Input: dimensioned drawing with shaded views. Units: mm. Origin: part minimum x, y, z. A direction names the side the tool comes from. Round coordinates to 2 decimals unless told otherwise and drop trailing zeros. Loops run counter-clockwise (first coordinate to the right, second up) from the corner with the lowest first, then second, coordinate; pieces in that order, holes last. Notation, with made-up numbers: (65, -18) - (112, -18) arc R17 ccw to (112, 10) - close; hole circle Ø11 at (71, 55). An arc over 180 degrees is marked (long way). Use CSV: the item, a comma, the result in double quotes. Start each with the question number.
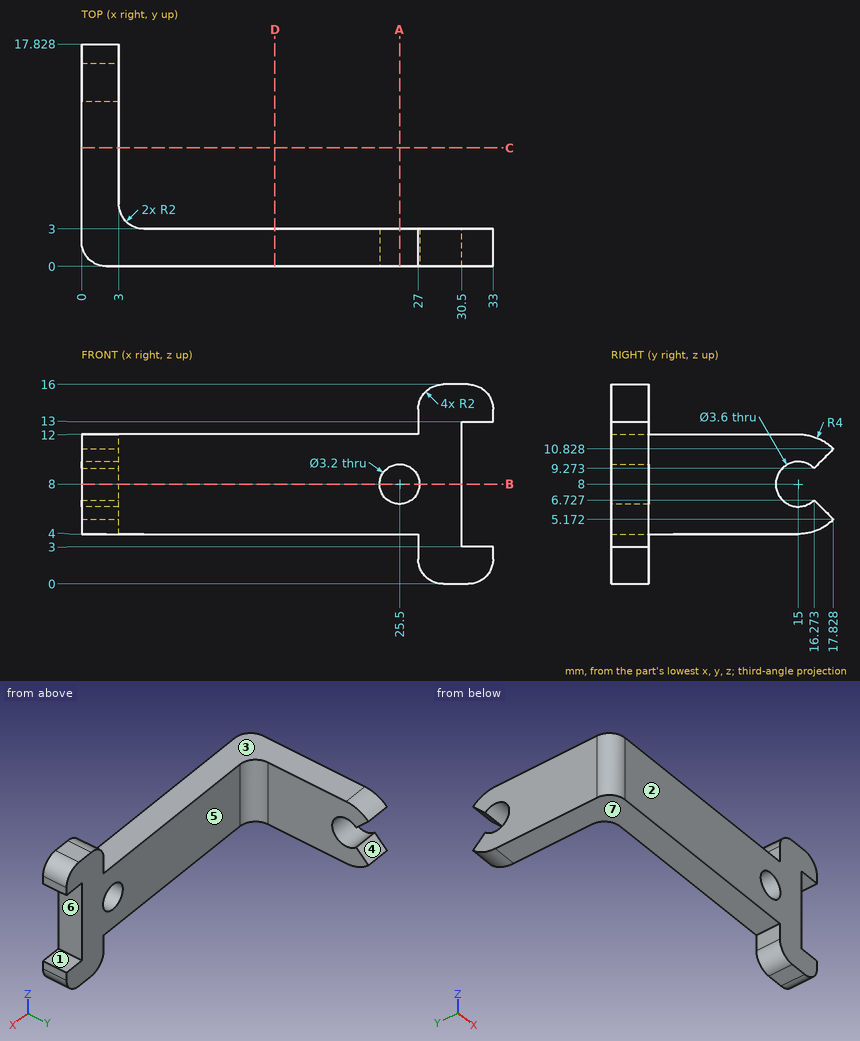
1. Mould query, pull axis Z, two halves, no side actions, for the marked faces 1, 2 and 3. Classes: +Z half, -Z half, draft (parallel to the pull), parting line (faces both ways), or undercut.
2. Section query B-B on z = 8. Return the cut outline in (x, y).
3. Section query A-A on x = 25.5. Return the cut outline in (y, z), and give its area (3 significant figures).
4. Section query C-C on y = 9.5. Return the cut outline in (x, z), and give its area (3 significant figures).
5. Line query: line 1 along X through (y, z) = (2.1, 8); line 2 along X through (y, z) = (2.25, 6); line 3 along Y through (x, z) = (5.5, 10.5). Output: solid intervals per line, ascending.
6. Reachability of the marked faces 4, 5, 6 and 7 from +Z, -Z, +X, -X, +Y, -Y: full face, straight path, thin tool, end or side. Return the list, or none.
7. Contact query for flat-ended pins moving along their axis: P1, Ø4, axis at x = 25.5, z = 8, coming from the +Y side; P2, Ø4, axis at y = 9.5, z = 9.5, coming from the +X side; P3, Ø1.2, axis at x = 32, y = 1, coming from the -Z side. Output: stop coordinate, or through.
Values:
1,face 1,"undercut"
1,face 2,"draft"
1,face 3,"+Z half"
2,outline,"(0, 2) arc R2 ccw to (2, 0) - (23.9, 0) - (23.9, 3) - (5, 3) arc R2 cw to (3, 5) - (3, 13.2) - (0, 13.2) - close; (27.1, 0) - (30.5, 0) - (30.5, 3) - (27.1, 3) - close"
3,outline,"(0, 4) - (3, 4) - (3, 6.4) - (0, 6.4) - close; (0, 9.6) - (3, 9.6) - (3, 12) - (0, 12) - close"
3,area,"14.4 mm^2"
4,outline,"(0, 4) - (3, 4) - (3, 12) - (0, 12) - close"
4,area,"24.0 mm^2"
5,line 1,"x = 0 to 23.9, 27.1 to 30.5"
5,line 2,"x = 0 to 30.5"
5,line 3,"y = 0 to 3"
6,face 4,"+X, -X, +Y"
6,face 5,"+Z, -Z, +X, +Y"
6,face 6,"+X, +Y, -Y"
6,face 7,"-Z, -X, +Y, -Y"
7,P1,"stops at y = 3"
7,P2,"stops at x = 3"
7,P3,"stops at z = 0.04"
